Could you check a few things on this drawing? It's one solid part, dimensions in mm from its lowest x, y, z. A direction names the side the tool comes from. Coordinates: 2 decimals unless noted, no trailing zeros. Loops run counter-clockwise (first coordinate to the right, second up) from the corner with the lowest first, then second, coordinate; pieces in that order, holes last. Notation, with made-up numbers: (-19.75, 11.5) -> (31.25, 11.5) arc R14 cw to (31.25, 30.5) -> close; hole circle Ø11 at (80.25, 11.5). An arc over 180 degrees is marked (long way). One line per question, with ' | ' between items.
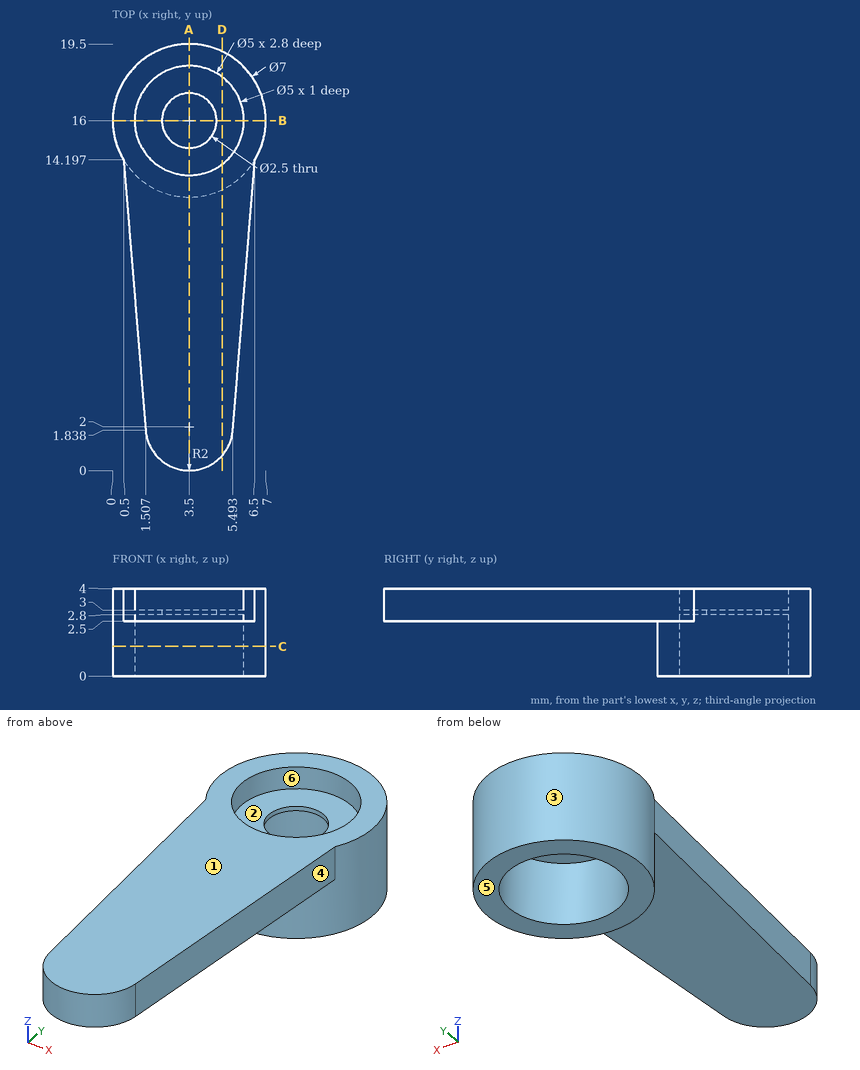
1) I need wall thicknesses on line 1 along Y through (x, z) = (3.5, 3.65); line 2 along Z through (x, y) = (5.5, 16.5); line 3 along Z through (x, y) = (4.75, 4.5). Which ranges of each line are inside material? Lowest first, please. Write a range as from..to.
Data:
line 1: 0..13.5, 18.5..19.5 | line 2: 2.8..3 | line 3: 2.5..4
2) If we section it at B-B on y = 16: Please give me the cut outline in (x, z).
Data:
outline: (0, 0) -> (1, 0) -> (1, 2.8) -> (2.25, 2.8) -> (2.25, 3) -> (1, 3) -> (1, 4) -> (0, 4) -> close; (4.75, 2.8) -> (6, 2.8) -> (6, 0) -> (7, 0) -> (7, 4) -> (6, 4) -> (6, 3) -> (4.75, 3) -> close
3) If we section it at A-A on x = 3.5: Please give me the cut outline in (y, z).
Data:
outline: (0, 2.5) -> (12.5, 2.5) -> (12.5, 0) -> (13.5, 0) -> (13.5, 2.8) -> (14.75, 2.8) -> (14.75, 3) -> (13.5, 3) -> (13.5, 4) -> (0, 4) -> close; (17.25, 2.8) -> (18.5, 2.8) -> (18.5, 0) -> (19.5, 0) -> (19.5, 4) -> (18.5, 4) -> (18.5, 3) -> (17.25, 3) -> close
4) If we section it at C-C on z = 1.35: Please give me the cut outline in (x, y).
Data:
outline: circle Ø7 at (3.5, 16); hole circle Ø5 at (3.5, 16)
5) If we section it at D-D on x = 5: Please give me the cut outline in (y, z).
Data:
outline: (0.68, 2.5) -> (12.84, 2.5) -> (12.84, 0) -> (14, 0) -> (14, 2.8) -> (18, 2.8) -> (18, 0) -> (19.16, 0) -> (19.16, 4) -> (18, 4) -> (18, 3) -> (14, 3) -> (14, 4) -> (0.68, 4) -> close
6) I'm going to push flat-ended pins straight in: pin 1 Ø4 at (x, y) = (3.5, 16) entering from +Z; pin 2 Ø2.5 at (x, y) = (4, 16) entering from -Z. Where does each tip first touch, or does it pass through?
Data:
pin 1: z = 3 | pin 2: z = 2.8
7) We'd pull the mould along X, two halves only. Please class the marked faces 4, 5 and 6: pulls with the +X half, pulls with the -X half, needs draft (parallel to the pull), parting line crosses it, or undercut.
Data:
face 4: pulls with the +X half | face 5: needs draft | face 6: undercut
8) On a 3-axis mill with a long thin cutter (end or side, diameter ignored), from which of +Z, -Z, +X, -X, +Y, -Y can I reach the whole of each face in a straight line? I mean the marked faces 1, 2 and 3. Say none if no direction works.
Data:
face 1: +Z, +X, -X, +Y, -Y | face 2: +Z | face 3: -Z
